```python
from build123d import *

# Parameters (mm, degrees)
ESQUISSE1_W              = 50
ESQUISSE1_H              = 31.5
ESQUISSE1_R              = 2.1
BOSS_EXTRU_1_DEPTH       = 8
ESQUISSE3_W              = 44
ESQUISSE3_H              = 31.5
BOSS_EXTRU_2_DEPTH       = 30
ESQUISSE4_R              = 8
ENL_V_MAT_EXTRU_1_DEPTH  = 60
ENL_V_MAT_EXTRU_2_DEPTH  = 56
ESQUISSE7_R              = 3.6
ENL_V_MAT_EXTRU_3_DEPTH  = 2
D_GAGEMENT_M51_D         = 5.3
D_GAGEMENT_M51_DEPTH     = 34
D_GAGEMENT_M51_TIP       = 1.59228064
ENL_V_MAT_EXTRU_4_DEPTH  = 8
ESQUISSE13_W             = 30
ESQUISSE13_H             = 22
ENL_V_MAT_EXTRU_6_DEPTH  = 58
ESQUISSE14_R             = 4
ENL_V_MAT_EXTRU_7_DEPTH  = 3
ESQUISSE15_R             = 1.25
ENL_V_MAT_EXTRU_8_DEPTH  = 5
BOSS_EXTRU_3_DEPTH       = 2
BOSS_EXTRU_4_START       = 2
ESQUISSE17_R             = 4
BOSS_EXTRU_4_DEPTH       = 2
ESQUISSE18_R             = 2.6
ENL_V_MAT_EXTRU_9_DEPTH  = 22
ESQUISSE19_R             = 4.25
ENL_V_MAT_EXTRU_10_DEPTH = 2


with BuildPart() as part:
    # Esquisse1 → Boss.-Extru.1 (new body)
    with BuildSketch(Plane.XY):
        with Locations((0, -15.75)):
            Rectangle(ESQUISSE1_W, ESQUISSE1_H)
        with Locations((17.5, -27.75)):
            Circle(ESQUISSE1_R, mode=Mode.SUBTRACT)
        with Locations((17.5, -3.75)):
            Circle(ESQUISSE1_R, mode=Mode.SUBTRACT)
        with Locations((-17.5, -3.75)):
            Circle(ESQUISSE1_R, mode=Mode.SUBTRACT)
        with Locations((-17.5, -27.75)):
            Circle(ESQUISSE1_R, mode=Mode.SUBTRACT)
    extrude(amount=BOSS_EXTRU_1_DEPTH)

    # Esquisse3 → Boss.-Extru.2 (add)
    with BuildSketch(Plane.ZY.offset(25)):
        with Locations((-14, -15.75)):
            Rectangle(ESQUISSE3_W, ESQUISSE3_H)
    extrude(amount=BOSS_EXTRU_2_DEPTH)

    # Esquisse4 → Enlèv. mat.-Extru.1 (cut)
    with BuildSketch(Plane.XY.offset(8)):
        with Locations((-36.7, -15.75)):
            Circle(ESQUISSE4_R)
    extrude(amount=-ENL_V_MAT_EXTRU_1_DEPTH, mode=Mode.SUBTRACT)

    # Esquisse6 → Enlèv. mat.-Extru.2 (cut)
    with BuildSketch(Plane.XY.offset(8)):
        with BuildLine():
            Line((-55, -14.5), (-44.601740315, -14.5))
            ThreePointArc((-44.601740315, -14.5), (-44.7, -15.75), (-44.601740315, -17))
            Line((-44.601740315, -17), (-55, -17))
            Line((-55, -17), (-55, -14.5))
        make_face()
    extrude(amount=-ENL_V_MAT_EXTRU_2_DEPTH, mode=Mode.SUBTRACT)

    # Esquisse7 → Enlèv. mat.-Extru.3 (cut)
    with BuildSketch(Plane.XY.offset(8)):
        with Locations((-17.5, -3.75)):
            Circle(ESQUISSE7_R)
        with Locations((-17.5, -27.75)):
            Circle(ESQUISSE7_R)
        with Locations((17.5, -27.75)):
            Circle(ESQUISSE7_R)
        with Locations((17.5, -3.75)):
            Circle(ESQUISSE7_R)
    extrude(amount=-ENL_V_MAT_EXTRU_3_DEPTH, mode=Mode.SUBTRACT)

    # Dégagement M51
    with Locations(Plane(origin=(0, 0, 0), x_dir=(1, 0, 0), z_dir=(0, 1, 0))):
        with Locations((-49, 2)):
            Hole(D_GAGEMENT_M51_D / 2, depth=D_GAGEMENT_M51_DEPTH)
            with Locations((0, 0, -(D_GAGEMENT_M51_DEPTH + D_GAGEMENT_M51_TIP / 2))):  # 118° drill point
                Cone(0, D_GAGEMENT_M51_D / 2, D_GAGEMENT_M51_TIP, mode=Mode.SUBTRACT)

    # Esquisse12 → Enlèv. mat.-Extru.4 (cut)
    with BuildSketch(Plane.XZ.offset(31.5)):
        Polygon((-45, 0.309401077), (-49, 2.618802154), (-53, 0.309401077), (-53, -4.309401077), (-49, -6.618802154), (-45, -4.309401077), align=None)
    extrude(amount=-ENL_V_MAT_EXTRU_4_DEPTH, mode=Mode.SUBTRACT)

    # Esquisse13 → Enlèv. mat.-Extru.6 (cut)
    with BuildSketch(Plane.XZ.offset(31.5)):
        with Locations((-40, -25)):
            Rectangle(ESQUISSE13_W, ESQUISSE13_H)
    extrude(amount=-ENL_V_MAT_EXTRU_6_DEPTH, mode=Mode.SUBTRACT)

    # Esquisse14 → Enlèv. mat.-Extru.7 (cut)
    with BuildSketch(Plane(origin=(0, 0, 0), x_dir=(1, 0, 0), z_dir=(0, 1, 0))):
        with Locations(Location((-49, 2, 0), (0, 0, 180))):
            Circle(ESQUISSE14_R)
    extrude(amount=-ENL_V_MAT_EXTRU_7_DEPTH, mode=Mode.SUBTRACT)

    # Esquisse15 → Enlèv. mat.-Extru.8 (cut)
    with BuildSketch(Plane.ZY.offset(55)):
        with Locations(Location((4, -20.5, 0), (0, 0, 270))):
            Circle(ESQUISSE15_R)
    extrude(amount=-ENL_V_MAT_EXTRU_8_DEPTH, mode=Mode.SUBTRACT)

    # Esquisse16 → Boss.-Extru.3 (add)
    with BuildSketch(Plane.XZ.offset(31.5)):
        Polygon((-55, 8), (-55, -14), (-25, -14), (-25, 0), (25, 0), (25, 8), align=None)
        Polygon((-53, 0.309401077), (-53, -4.309401077), (-49, -6.618802154), (-45, -4.309401077), (-45, 0.309401077), (-49, 2.618802154), align=None, mode=Mode.SUBTRACT)
    extrude(amount=BOSS_EXTRU_3_DEPTH)

    # Esquisse17 → Boss.-Extru.4 (add)
    with BuildSketch(Plane(origin=(0, 0, 0), x_dir=(1, 0, 0), z_dir=(0, 1, 0)).offset(BOSS_EXTRU_4_START)):
        Polygon((-25, 0), (-25, 14), (-55, 14), (-55, -8), (25, -8), (25, 0), align=None)
        with Locations(Location((-49, 2, 0), (0, 0, 180))):
            Circle(ESQUISSE17_R, mode=Mode.SUBTRACT)
    extrude(amount=-BOSS_EXTRU_4_DEPTH)

    # Esquisse18 → Enlèv. mat.-Extru.9 (cut)
    with BuildSketch(Plane.XY.offset(8)):
        with Locations((-17.5, -3.75)):
            Circle(ESQUISSE18_R)
        with Locations((17.5, -3.75)):
            Circle(ESQUISSE18_R)
        with Locations((17.5, -27.75)):
            Circle(ESQUISSE18_R)
        with Locations((-17.5, -27.75)):
            Circle(ESQUISSE18_R)
    extrude(amount=-ENL_V_MAT_EXTRU_9_DEPTH, mode=Mode.SUBTRACT)

    # Esquisse19 → Enlèv. mat.-Extru.10 (cut)
    with BuildSketch(Plane.XY.offset(8)):
        with Locations((-17.5, -3.75)):
            Circle(ESQUISSE19_R)
        with Locations((17.5, -3.75)):
            Circle(ESQUISSE19_R)
        with Locations((17.5, -27.75)):
            Circle(ESQUISSE19_R)
        with Locations((-17.5, -27.75)):
            Circle(ESQUISSE19_R)
    extrude(amount=-ENL_V_MAT_EXTRU_10_DEPTH, mode=Mode.SUBTRACT)


solid = part.part
```
Source: CAD feature listing. Evaluate the final solid. Frame: model axes, mm. A direction names the side the tool comes from. Coordinates: 2 decimals unless noted, no trailing zeros. Loops run counter-clockwise (first coordinate to the right, second up) from the corner with the lowest first, then second, coordinate; pieces in that order, holes last. Notation, with made-up numbers: M -35,-5.5 L -29,-5.5 A8 cw -29,3.5 Z; hole C 50,2 d10. An arc over 180 degrees is marked long. Use a Markdown table: item, result. Add a question column.
Q1. Material intervals for L1, parallel to Y at x = -17.5, z = 1.7; L2, parallel to Y at x = -47, z = -4.25; L3, parallel to X at y = -13, z = 0.25, sorted ascending.
Q2. Section query C-C, the plane z = -2. Return loops of the section in (x, y).
Q3. Draft query along Z for faces 6 (the cylindrical face through (19.98, -26.97, 3.04)), 7 (the flat face through (-50, -20, 4)), 8 (the flat face through (17, -31, 6)). Return one class per face: pulls with the +Z half, pulls with the -Z half, needs draft (parallel to the pull), parting line crosses it, or undercut.
Q4. Section query B-B, the plane y = -20.5. Return loops of the section in (x, z), and give its area (3 significant figures).
Q5. Section query D-D, the plane z = -9. Return loops of the section in (x, y).
Q6. First-contact query: pin 1 (7 mm diameter, centred on x = -17.5, y = -3.75, fed in from -Z); pin 2 (7 mm diameter, centred on x = -49, z = -2, fed in from -Y). Flat tips, straight axial feed; report the tip coordinate or a pass-through.
Q7. Section query A-A, the plane x = 17.5. Return loops of the section in (y, z).
Q8. Access query for faces 1 (the flat face through (-45, -28, -2)), 2 (the cylindrical face through (-45, 0, -2)), 3 (the flat face through (-52, -14.5, -3)), 4 (the flat face through (-18, -7, 6)), 5 (the flat face through (-25, -16, -7)). Directions: +Z, -Z, +X, -X, +Y, -Y. A direction counts if a zero-diameter tool reaches every point of the face in a straight line with its end or side. Return the directions, or none.
Result:
| question | item | result |
|---|---|---|
| 1 | L1 | y = -33.5 to -30.35, -25.15 to -6.35, -1.15 to 2 |
| 1 | L2 | y = -23.5 to -17, -14.5 to -3 |
| 1 | L3 | x = -55 to -50.4, -47.6 to -44.21, -29.19 to 25 |
| 2 | outline | M -55,-33.5 L -53,-33.5 L -53,-23.5 L -51.65,-23.5 L -51.65,-17 L -55,-17 Z; M -55,-14.5 L -51.65,-14.5 L -51.65,-3 L -53,-3 L -53,2 L -55,2 Z; M -46.35,-23.5 L -45,-23.5 L -45,-33.5 L -25,-33.5 L -25,2 L -45,2 L -45,-3 L -46.35,-3 L -46.35,-14.5 L -44.6,-14.5 A8 cw long -44.6,-17 L -46.35,-17 Z |
| 3 | face 6 | needs draft |
| 3 | face 7 | undercut |
| 3 | face 8 | pulls with the +Z half |
| 4 | outline | M -55,-14 L -43.14,-14 L -43.14,8 L -55,8 L -55,5.25 L -50,5.25 L -50,2.75 L -55,2.75 Z; M -30.26,-14 L -25,-14 L -25,0 L 25,0 L 25,8 L -30.26,8 Z; hole C -49,-2 d5.3 |
| 4 | area | 742 mm2 |
| 5 | outline | M -55,-33.5 L -25,-33.5 L -25,2 L -55,2 L -55,-14.5 L -44.6,-14.5 A8 cw long -44.6,-17 L -55,-17 Z |
| 6 | pin 1 | stops at z = 0 |
| 6 | pin 2 | stops at y = -23.5 |
| 7 | outline | M -33.5,0 L -30.35,0 L -30.35,6 L -32,6 L -32,8 L -33.5,8 Z; M -25.15,0 L -6.35,0 L -6.35,6 L -8,6 L -8,8 L -23.5,8 L -23.5,6 L -25.15,6 Z; M -1.15,0 L 2,0 L 2,8 L 0.5,8 L 0.5,6 L -1.15,6 Z |
| 8 | face 1 | -Y |
| 8 | face 2 | +Y |
| 8 | face 3 | +Z, -Z, -X |
| 8 | face 4 | +Z |
| 8 | face 5 | -Z, +X, +Y, -Y |
